The listing builds one solid part. Answer for the finished solid, in the listing's coordinates (mm). Face numbers are marked on the shaded views. A direction names the side the tool comes from. Coordinates: 2 decimals unless noted, no trailing zeros. Loops run counter-clockwise (first coordinate to the right, second up) from the corner with the lowest first, then second, coordinate; pieces in that order, holes last. Notation, with made-up numbers: (62.5, 18.25) -> (102.5, 18.25) arc R10 cw to (102.5, 25.25) -> close; hole circle Ø3 at (70.5, -9.75). An arc over 180 degrees is marked (long way). Answer in a Markdown table with one row per item.
```python
from build123d import *

# Parameters (mm, degrees)
SKETCH1_W           = 86
SKETCH1_H           = 23
BOSS_EXTRUDE1_DEPTH = 3.175
BOSS_EXTRUDE2_DEPTH = 3.175
RIB4_REACH          = 68.401
SKETCH11_WALL_W     = 152.68434621
SKETCH11_WALL_H     = 2.54
SKETCH17_W          = 12.7
SKETCH17_H          = 10.795
CUT_EXTRUDE1_DEPTH  = 50.945290319
SKETCH18_R          = 2.159
CUT_EXTRUDE2_DEPTH  = 127
SKETCH19_R          = 1.397
CUT_EXTRUDE3_DEPTH  = 47.652019249
SKETCH21_W          = 1.27
SKETCH21_H          = 10.795
CUT_EXTRUDE4_DEPTH  = 50.945290319
SKETCH23_W          = 57.219873646
SKETCH23_H          = 16.240764414
SKETCH23_W_2        = 21.450294578
SKETCH23_H_2        = 16.117794019
CUT_EXTRUDE5_DEPTH  = 47.652019249


with BuildPart() as part:
    # Sketch1 → Boss-Extrude1 (new body)
    with BuildSketch(Plane.XY):
        Rectangle(SKETCH1_W, SKETCH1_H)
    extrude(amount=-BOSS_EXTRUDE1_DEPTH)

    # Sketch3 → Boss-Extrude2 (add)
    with BuildSketch(Plane(origin=(0, -11.5, 0), x_dir=(-1, 0, 0), z_dir=(0, -1, 0))):
        Polygon((34.200000011, 0), (34.200000011, -10.795), (8.80000001, -10.795), (8.800000011, 0), align=None)
        Polygon((-34.200000011, 0), (-34.200000011, -10.795), (-8.80000001, -10.795), (-8.800000011, 0), align=None)
    extrude(amount=-BOSS_EXTRUDE2_DEPTH)

    # Sketch11 wall → Rib4 (add, up to next)
    with BuildSketch(Plane(origin=(-21.500000011, -0.407189587, 4.154640606), x_dir=(-5.6e-11, -0.885499596527, 0.46464014522), z_dir=(0, 0.46464014522, 0.885499596527)), mode=Mode.PRIVATE) as rib4_sk1:
        Rectangle(SKETCH11_WALL_W, SKETCH11_WALL_H)
    rib4_tool1 = extrude(rib4_sk1.sketch, amount=-RIB4_REACH, mode=Mode.PRIVATE) - part.part
    rib4 = rib4_tool1.solids().sort_by_distance((-21.500000011, -0.407189587, 4.154640606))[0]
    add(rib4)

    # Mirror1: Rib4 across plane
    add(rib4.mirror(Plane(origin=(0, 0, 0), x_dir=(0, 0, 1), z_dir=(1, 0, 0))))

    # Sketch17 → Cut-Extrude1 (cut, through all)
    with BuildSketch(Plane(origin=(0, 11.5, 0), x_dir=(1, 0, 0), z_dir=(0, 1, 0))):
        with Locations((-15.15000001, -5.3975)):
            Rectangle(SKETCH17_W, SKETCH17_H)
        with Locations((27.850000011, -5.3975)):
            Rectangle(SKETCH17_W, SKETCH17_H)
    extrude(amount=-CUT_EXTRUDE1_DEPTH, mode=Mode.SUBTRACT)

    # Sketch18 → Cut-Extrude2 (cut)
    with BuildSketch(Plane(origin=(0, 11.5, 0), x_dir=(1, 0, 0), z_dir=(0, 1, 0))):
        with Locations(Location((-28.373739812, -5.177433052, 0), (0, 0, 270))):
            Circle(SKETCH18_R)
        with Locations(Location((14.806260188, -5.177433052, 0), (0, 0, 90))):
            Circle(SKETCH18_R)
    extrude(amount=-CUT_EXTRUDE2_DEPTH, mode=Mode.SUBTRACT)

    # Sketch19 → Cut-Extrude3 (cut, through all)
    with BuildSketch(Plane(origin=(0, 0, -3.175), x_dir=(-1, 0, 0), z_dir=(0, 0, -1))):
        with Locations((-39.952, -8.452)):
            Circle(SKETCH19_R)
        with Locations((-17.473, 8.7438)):
            Circle(SKETCH19_R)
        with Locations((17.9429, -6.801)):
            Circle(SKETCH19_R)
        with Locations((40.206, -8.579)):
            Circle(SKETCH19_R)
    extrude(amount=-CUT_EXTRUDE3_DEPTH, mode=Mode.SUBTRACT)

    # Sketch21 → Cut-Extrude4 (cut, through all)
    with BuildSketch(Plane(origin=(0, 11.5, 0), x_dir=(1, 0, 0), z_dir=(0, 1, 0))):
        with Locations((-22.13500001, -5.3975)):
            Rectangle(SKETCH21_W, SKETCH21_H)
    extrude(amount=-CUT_EXTRUDE4_DEPTH, mode=Mode.SUBTRACT)

    # Sketch23 → Cut-Extrude5 (cut, through all)
    with BuildSketch(Plane(origin=(0, 0, -3.175), x_dir=(-1, 0, 0), z_dir=(0, 0, -1))):
        with Locations((14.390063177, 3.379617793)):
            Rectangle(SKETCH23_W, SKETCH23_H)
        with Locations((-32.274852711, 3.44110299)):
            Rectangle(SKETCH23_W_2, SKETCH23_H_2)
    extrude(amount=-CUT_EXTRUDE5_DEPTH, mode=Mode.SUBTRACT)


solid = part.part
```
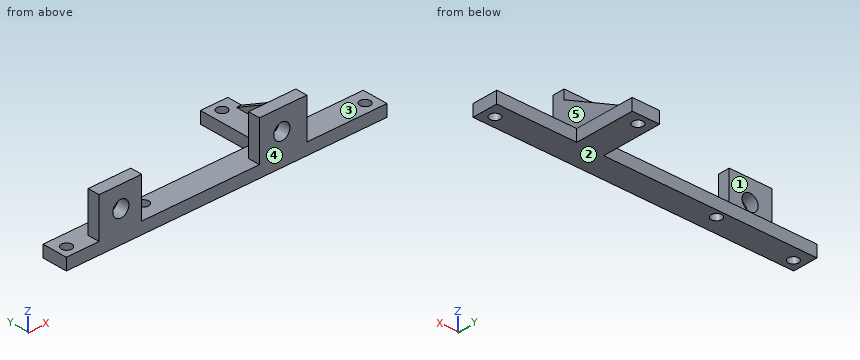
Item 1: A tool of negligible diameter and unlimited length cuts with its end or side. For the marked faces 1 and 2, from which of +Z, -Z, +X, -X, +Y, -Y can it reach the whole face along a straight path? Write none if from no direction.
Findings below:
| item | result |
|---|---|
| face 1 | +Z, -X, +Y |
| face 2 | -Z, +X, -X, +Y, -Y |
Item 2: A cutting plane is placed at C-C, the plane x = -18. Determine the outline of the cut face in (y, z) (3 decimals).
Findings below:
| item | result |
|---|---|
| outline | (-11.5, -3.175) -> (-8.197, -3.175) -> (-8.197, 0) -> (-11.5, 0) -> close; (-5.405, -3.175) -> (-4.741, -3.175) -> (-4.741, 0) -> (-5.405, 0) -> close |
Item 3: Find the intervals of material crossed by probe 1 along X at (y, z) = (-10, 2.25); probe 2 along X at (y, z) = (-10, 4); probe 3 along X at (y, z) = (-7, -1.5), in increasing order.
Findings below:
| item | result |
|---|---|
| probe 1 | x = -34.2 to -22.77, 8.8 to 21.5 |
| probe 2 | x = -34.2 to -30.18, -26.56 to -22.77, 8.8 to 13, 16.62 to 21.5 |
| probe 3 | x = -43 to -19.33, -16.56 to 43 |
Item 4: A cutting plane is placed at A-A, the plane z = 9.5. Determine the outline of the cut face in (x, y) (3 decimals), plus the area to 3 significant figures.
Findings below:
| item | result |
|---|---|
| outline | (-34.2, -11.5) -> (-22.77, -11.5) -> (-22.77, -8.325) -> (-34.2, -8.325) -> close; (8.8, -11.5) -> (21.5, -11.5) -> (21.5, -8.325) -> (8.8, -8.325) -> close |
| area | 76.6 mm2 |
Item 5: A cutting plane is placed at D-D, the plane z = -1.25. Determine the outline of the cut face in (x, y) (3 decimals), plus the area to 3 significant figures.
Findings below:
| item | result |
|---|---|
| outline | (-43, -11.5) -> (43, -11.5) -> (43, -4.618) -> (21.55, -4.618) -> (21.55, 11.5) -> (14.22, 11.5) -> (14.22, -4.741) -> (-43, -4.741) -> close; hole circle Ø2.794 at (-40.206, -8.579); hole circle Ø2.794 at (-17.943, -6.801); hole circle Ø2.794 at (17.473, 8.744); hole circle Ø2.794 at (39.952, -8.452) |
| area | 678 mm2 |
Item 6: Flat-ended cylindrical pins translate along their axes: pin 1 Ø2.5 at (y, z) = (2.5, -2) entering from +X; pin 2 Ø5.5 at (x, z) = (-28.37, 5.18) entering from +Y (3 decimals); pin 3 Ø3.5 at (x, y) = (17.47, 8.74) entering from +Z. Find the tip coordinate at first contact, or state that the pin passes through.
Findings below:
| item | result |
|---|---|
| pin 1 | stops at x = 21.55 |
| pin 2 | stops at y = -8.325 |
| pin 3 | stops at z = 0 |
Item 7: A cutting plane is placed at B-B, the plane z = 4.75. Determine the outline of the cut face in (x, y) (3 decimals).
Findings below:
| item | result |
|---|---|
| outline | (-34.2, -11.5) -> (-30.49, -11.5) -> (-30.49, -8.325) -> (-34.2, -8.325) -> close; (-26.257, -11.5) -> (-22.77, -11.5) -> (-22.77, -8.325) -> (-26.257, -8.325) -> close; (8.8, -11.5) -> (12.69, -11.5) -> (12.69, -8.325) -> (8.8, -8.325) -> close; (16.923, -11.5) -> (21.5, -11.5) -> (21.5, -1.542) -> (20.23, -1.542) -> (20.23, -8.325) -> (16.923, -8.325) -> close |
Item 8: Determine the mould class of the marked faces 3, 4 and 5 for opening direction X: +X half, -X half, draft (parallel to the pull), parting line (faces both ways), or undercut.
Findings below:
| item | result |
|---|---|
| face 3 | undercut |
| face 4 | draft |
| face 5 | +X half |
